Autodesk Inventor part; units mm, degrees
ref_plane "YZ Plane" through (0, 0, 0) normal (1, 0, 0) x (0, 1, 0)
ref_plane "XZ Plane" through (0, 0, 0) normal (0, 1, 0) x (-1, 0, 0)
ref_plane "XY Plane" through (0, 0, 0) normal (0, 0, 1) x (1, 0, 0)
sketch "Sketch1" plane through (0, 0, 0) normal (0, 0, 1) x (1, 0, 0)
  line L0 (6.35, 0) -> (120.65, 0)
  line L1 (127, 6.35) -> (127, 31.75)
  line L2 (120.65, 38.1) -> (107.95, 38.1)
  line L3 (101.6, 44.45) -> (101.6, 95.25)
  line L4 (95.25, 101.6) -> (31.75, 101.6)
  line L5 (25.4, 95.25) -> (25.4, 44.45)
  line L6 (19.05, 38.1) -> (6.35, 38.1)
  line L7 (0, 31.75) -> (0, 6.35)
  arc A0 (31.75, 101.6) -> (25.4, 95.25) centre (31.75, 95.25) ccw
  arc A1 (19.05, 38.1) -> (25.4, 44.45) centre (19.05, 44.45) ccw
  arc A2 (6.35, 38.1) -> (0, 31.75) centre (6.35, 31.75) ccw
  arc A3 (0, 6.35) -> (6.35, 0) centre (6.35, 6.35) ccw
  arc A4 (120.65, 0) -> (127, 6.35) centre (120.65, 6.35) ccw
  arc A5 (127, 31.75) -> (120.65, 38.1) centre (120.65, 31.75) ccw
  arc A6 (101.6, 44.45) -> (107.95, 38.1) centre (107.95, 44.45) ccw
  arc A7 (101.6, 95.25) -> (95.25, 101.6) centre (95.25, 95.25) ccw
  line L8 (57.15, 50.8) -> (69.85, 50.8)
  line L9 (76.2, 57.15) -> (76.2, 82.55)
  line L10 (69.85, 88.9) -> (57.15, 88.9)
  line L11 (50.8, 82.55) -> (50.8, 57.15)
  arc A8 (38.1, 25.4) -> (38.1, 12.7) centre (38.1, 19.05) ccw
  arc A9 (88.9, 12.7) -> (88.9, 25.4) centre (88.9, 19.05) ccw
  line L12 (38.1, 25.4) -> (88.9, 25.4)
  line L13 (88.9, 12.7) -> (38.1, 12.7)
  arc A10 (57.15, 88.9) -> (50.8, 82.55) centre (57.15, 82.55) ccw
  arc A11 (50.8, 57.15) -> (57.15, 50.8) centre (57.15, 57.15) ccw
  arc A12 (69.85, 50.8) -> (76.2, 57.15) centre (69.85, 57.15) ccw
  arc A13 (76.2, 82.55) -> (69.85, 88.9) centre (69.85, 82.55) ccw
  point P0 (0, 0)
  point P1 (127, 0)
  point P2 (127, 38.1)
  point P3 (101.6, 38.1)
  point P4 (25.4, 38.1)
  point P5 (0, 38.1)
  dimension "d0" = 127
  dimension "d1" = 38.1
  dimension "d2" = 25.4
  dimension "d3" = 6.35
  dimension "d4" = 6.35
extrude "Extrusion1" add sketch "Sketch1" along normal blind 9.525
properties part number "P2-7"
Can you work these out from the model? Positions are in its coordinate system, mm. A direction names the side the tool comes from. Coordinates: 2 decimals unless noted, no trailing zeros. Loops run counter-clockwise (first coordinate to the right, second up) from the corner with the lowest first, then second, coordinate; pieces in that order, holes last. Notation, with made-up numbers: (20.25, 83.25) - (61.25, 83.25) arc R19 ccw to (61.25, 115.25) - close; hole circle Ø1 at (30.5, -20.75). An arc over 180 degrees is marked (long way). Answer as CSV lines item,"result". Start each with the question number.
1) Suppose I cut it at C-C (z = 3.75). Please give me the cut outline in (x, y), plus the area to 3 significant figures.
2) Suppose I cut it at D-D (y = 19.05). Please give me the cut outline in (x, z) (3 decimals), plus the area to 3 significant figures.
3) Thinking about a two-plate mould opening in X: for faces 4 (the cylindrical face through (1.91, 1.81, 4.7)), 5 (the cylindrical face through (74.29, 87.09, 4.7)), 6 (the flat face through (127, 19, 5)), 7 (the cylindrical face through (52.71, 52.61, 4.7)), which applies, pulls with the +X half, pulls with the -X half, needs draft (parallel to the pull), parting line crosses it, or undercut?
4) Suppose I cut it at A-A (y = 76). Please give me the cut outline in (x, z) (3 decimals), plus the area to 3 significant figures.
5) For pin 1 (3 mm diameter, centred on y = 74, z = 6.5, fed in from -X); pin 2 (5 mm diameter, centred on y = 66, z = 6.5, fed in from +X); pin 3 (3 mm diameter, centred on x = 14.5, z = 3.5, fed in from +Y), each with a flat end and sliding along its axis, tell me the tip position at first contact or that it passes through.
6) Suppose I cut it at B-B (x = 58.5). Please give me the cut outline in (y, z) (3 decimals).
7) I need wall thicknesses on line 1 (Y direction, x = 69.5, z = 5); line 2 (X direction, y = 57.5, z = 8.5); line 3 (Y direction, x = 121, z = 6.75). Which ranges of each line are inside material? Lowest first, please. Write a range as from..to.
8) Which directions (+Z, -Z, +X, -X, +Y, -Y) give clear straight access to the entire face, cutting with the end or side of a thin tool? Please do faces 1 (the flat face through (76.2, 70, 5)), 2 (the flat face through (114, 38.1, 5)), 3 (the flat face through (63, 0, 5)).
Check result:
1,outline,"(0, 6.35) arc R6.35 ccw to (6.35, 0) - (120.65, 0) arc R6.35 ccw to (127, 6.35) - (127, 31.75) arc R6.35 ccw to (120.65, 38.1) - (107.95, 38.1) arc R6.35 cw to (101.6, 44.45) - (101.6, 95.25) arc R6.35 ccw to (95.25, 101.6) - (31.75, 101.6) arc R6.35 ccw to (25.4, 95.25) - (25.4, 44.45) arc R6.35 cw to (19.05, 38.1) - (6.35, 38.1) arc R6.35 ccw to (0, 31.75) - close; hole (38.1, 12.7) - (88.9, 12.7) arc R6.35 ccw to (88.9, 25.4) - (38.1, 25.4) arc R6.35 ccw to start; hole (50.8, 57.15) arc R6.35 ccw to (57.15, 50.8) - (69.85, 50.8) arc R6.35 ccw to (76.2, 57.15) - (76.2, 82.55) arc R6.35 ccw to (69.85, 88.9) - (57.15, 88.9) arc R6.35 ccw to (50.8, 82.55) - close"
1,area,"7,940 mm²"
2,outline,"(0, 0) - (31.75, 0) - (31.75, 9.525) - (0, 9.525) - close; (95.25, 0) - (127, 0) - (127, 9.525) - (95.25, 9.525) - close"
2,area,"605 mm²"
3,face 4,"pulls with the -X half"
3,face 5,"undercut"
3,face 6,"pulls with the +X half"
3,face 7,"undercut"
4,outline,"(25.4, 0) - (50.8, 0) - (50.8, 9.525) - (25.4, 9.525) - close; (76.2, 0) - (101.6, 0) - (101.6, 9.525) - (76.2, 9.525) - close"
4,area,"484 mm²"
5,pin 1,"stops at x = 25.4"
5,pin 2,"stops at x = 101.6"
5,pin 3,"stops at y = 38.1"
6,outline,"(0, 0) - (12.7, 0) - (12.7, 9.525) - (0, 9.525) - close; (25.4, 0) - (50.8, 0) - (50.8, 9.525) - (25.4, 9.525) - close; (88.9, 0) - (101.6, 0) - (101.6, 9.525) - (88.9, 9.525) - close"
7,line 1,"y = 0..12.7, 25.4..50.8, 88.9..101.6"
7,line 2,"x = 25.4..50.8, 76.2..101.6"
7,line 3,"y = 0.01..38.09"
8,face 1,"+Z, -Z"
8,face 2,"+Z, -Z, +X, +Y"
8,face 3,"+Z, -Z, +X, -X, -Y"
